The drawing under review shows one solid part. Ordinate dimensions are in mm from its lowest x, y, z. Round coordinates to 2 decimals unless told otherwise and drop trailing zeros. Order: outer loops, then holes, each group sorted by start corner. A loop starts at its lowest first (then second) coordinate and runs counter-clockwise, first axis right, second up. Notation, with made-up numbers: (23.25, 61) -> (56.25, 61) arc R22 ccw to (56.25, 96) -> close; hole circle Ø11 at (19.25, 80.5). An arc over 180 degrees is marked (long way). Use a Markdown table: item, result. Add a question column.
1) Consider section B-B (y = 22). State the section outline as (x, z) points.
2) Wall thickness on line 1 along Z through (x, y) = (1.55, 47.5); line 2 along Z through (x, y) = (1.9, 23.5); line 3 along Y through (x, z) = (2.1, 56): over which ranges is each line inside the solid? List them lowest first. Write a range as [from, to].
3) Consider section A-A (z = 55). State the section outline as (x, y) points, plus the area to 3 significant figures.
4) Consider section C-C (z = 18). State the section outline as (x, y) points, plus the area to 3 significant figures.
5) Clearance check with flat-ended pins moving along their axes: P1, Ø1, axis at x = 1, z = 11.5, coming from the -Y side; P2, Ø1.5, axis at x = 1.5, z = 57, coming from the +Y side; P3, Ø1.5, axis at x = 2, z = 95, coming from the +Y side. State where each tip first meets the part, or that it passes through.
6) Consider section D-D (y = 43). State the section outline as (x, z) points, plus the area to 3 significant figures.
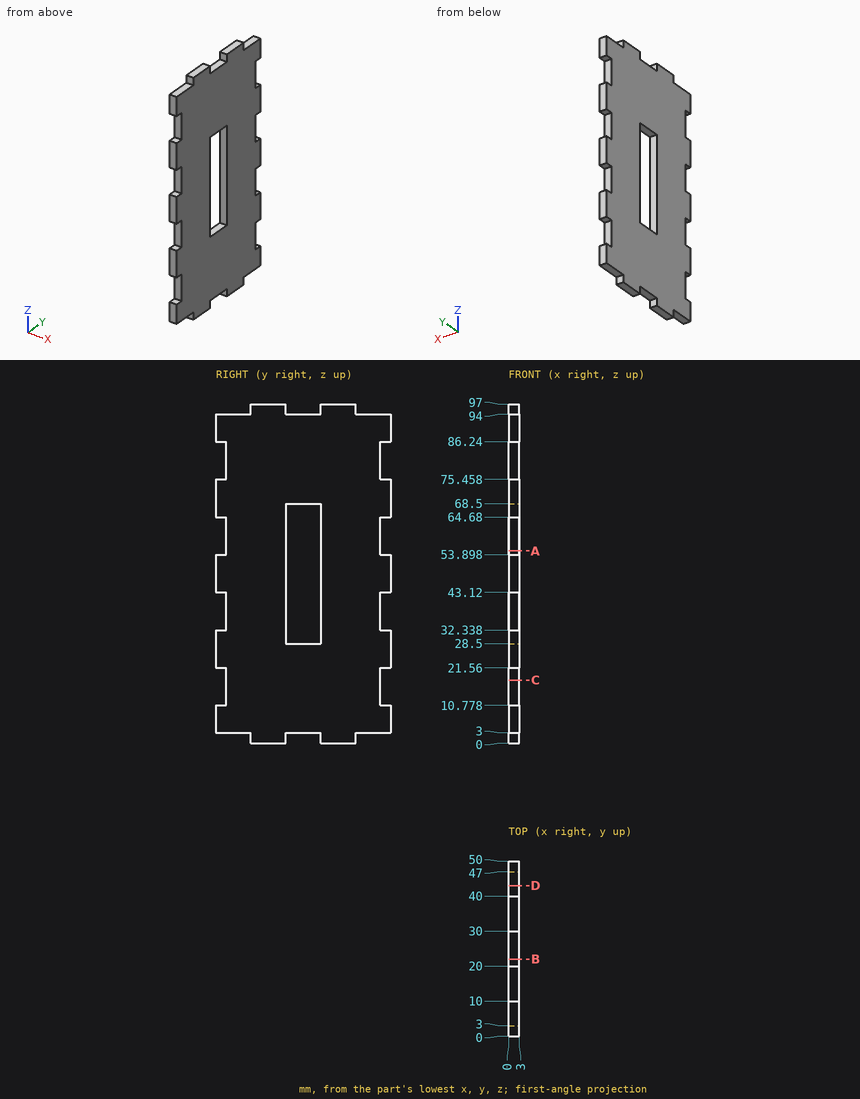
Results list:
| question | item | result |
|---|---|---|
| 1 | outline | (0, 3) -> (3, 3) -> (3, 28.5) -> (0, 28.5) -> close; (0, 68.5) -> (3, 68.5) -> (3, 94) -> (0, 94) -> close |
| 2 | line 1 | [3, 10.78], [21.56, 32.34], [43.12, 53.9], [64.68, 75.46], [86.24, 94] |
| 2 | line 2 | [3, 28.5], [68.5, 94] |
| 2 | line 3 | [3, 20], [30, 47] |
| 3 | outline | (0, 3) -> (3, 3) -> (3, 20) -> (0, 20) -> close; (0, 30) -> (3, 30) -> (3, 47) -> (0, 47) -> close |
| 3 | area | 102 mm2 |
| 4 | outline | (0, 3) -> (3, 3) -> (3, 47) -> (0, 47) -> close |
| 4 | area | 132 mm2 |
| 5 | P1 | y = 3 |
| 5 | P2 | y = 47 |
| 5 | P3 | y = 40 |
| 6 | outline | (0, 3) -> (3, 3) -> (3, 94) -> (0, 94) -> close |
| 6 | area | 273 mm2 |
